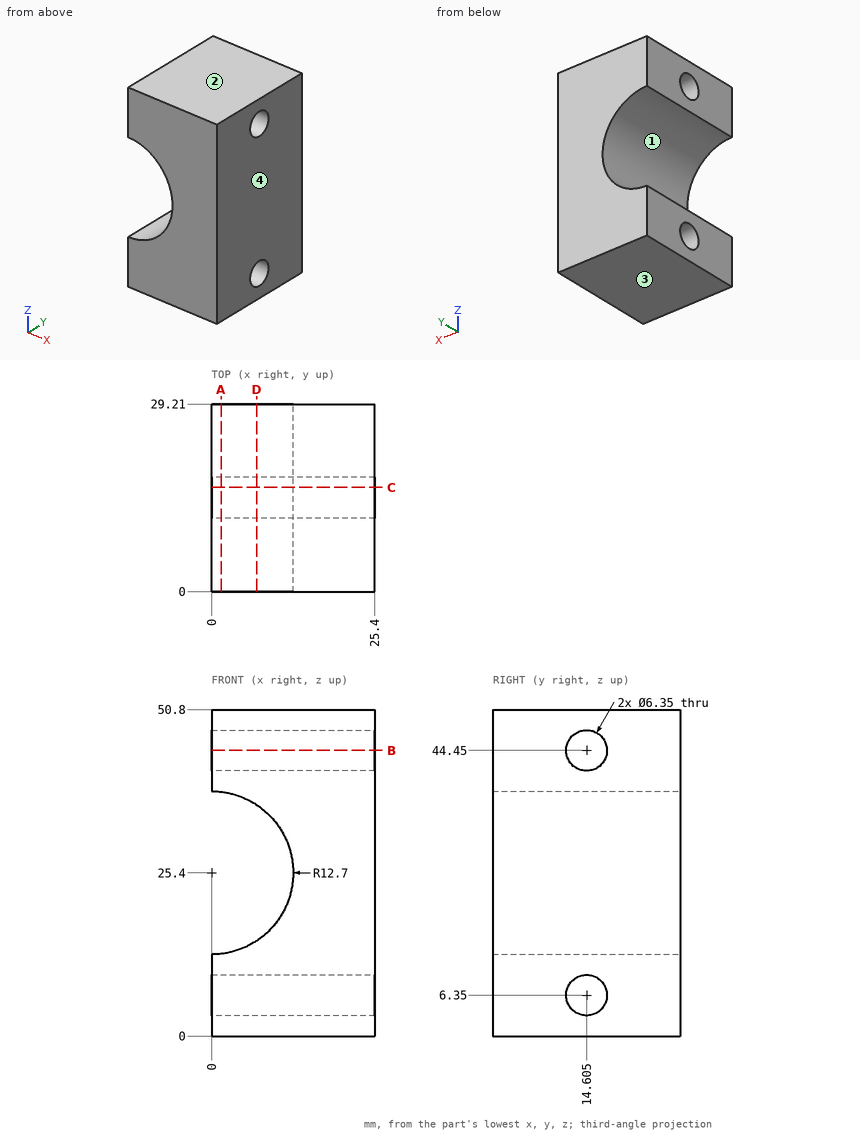
The drawing under review shows one solid part. Ordinate dimensions are in mm from its lowest x, y, z. Round coordinates to 2 decimals unless told otherwise and drop trailing zeros. Write each loop counter-clockwise with the first axis right and the second up, starting at its lowest first coordinate (ties: lowest second). Pieces come first, ordered by that corner, then holes. Notation, with made-up numbers: (13.5, 80) - (64.5, 80) arc R12 cw to (64.5, 101) - close; hole circle Ø1 at (-5.5, 74.25). An arc over 180 degrees is marked (long way). Put each result on its own line as item: value.
Q1. Mouldability with a two-part tool opening along Z and no side actions: class the marked faces 1, 2, 3 and 4 as released by +Z, released by -Z, zero draft, split by the parting line, or undercut.
Solved:
face 1: undercut
face 2: released by +Z
face 3: released by -Z
face 4: zero draft
Q2. We need section C-C (y = 16.25). Give the boundary of the cut face in (x, z).
Solved:
outline: (0, 0) - (25.4, 0) - (25.4, 3.63) - (0, 3.63) - close; (0, 9.07) - (25.4, 9.07) - (25.4, 41.73) - (0, 41.73) - (0, 38.1) arc R12.7 cw to (0, 12.7) - close; (0, 47.17) - (25.4, 47.17) - (25.4, 50.8) - (0, 50.8) - close
Q3. We need section D-D (x = 7). Give the boundary of the cut face in (y, z) (3 decimals), and give its area (3 significant figures).
Solved:
outline: (0, 0) - (29.21, 0) - (29.21, 14.803) - (0, 14.803) - close; (0, 35.997) - (29.21, 35.997) - (29.21, 50.8) - (0, 50.8) - close; hole circle Ø6.35 at (14.605, 6.35); hole circle Ø6.35 at (14.605, 44.45)
area: 801 mm2
Q4. Wall thickness on probe 1 along Z at (x, y) = (18.5, 13.75); probe 2 along Z at (x, y) = (18, 12.5); probe 3 along Z at (x, y) = (10, 14.5): over which ranges is each line inside the solid? List them lowest first.
Solved:
probe 1: z = 0 to 3.29, 9.41 to 41.39, 47.51 to 50.8
probe 2: z = 0 to 3.97, 8.73 to 42.07, 46.83 to 50.8
probe 3: z = 0 to 3.18, 9.52 to 17.57, 33.23 to 41.28, 47.62 to 50.8
Q5. We need section A-A (x = 1.5). Give the boundary of the cut face in (y, z) (3 decimals).
Solved:
outline: (0, 0) - (29.21, 0) - (29.21, 12.789) - (0, 12.789) - close; (0, 38.011) - (29.21, 38.011) - (29.21, 50.8) - (0, 50.8) - close; hole circle Ø6.35 at (14.605, 6.35); hole circle Ø6.35 at (14.605, 44.45)
Q6. We need section B-B (z = 44.45). Give the boundary of the cut face in (x, y), and give its area (3 significant figures).
Solved:
outline: (0, 0) - (25.4, 0) - (25.4, 11.43) - (0, 11.43) - close; (0, 17.78) - (25.4, 17.78) - (25.4, 29.21) - (0, 29.21) - close
area: 581 mm2
Q7. Insertion check: pin 1 Ø10 at (y, z) = (14.605, 44.45) entering from -X; pin 2 Ø1.5 at (y, z) = (23, 33.5) entering from -X; pin 3 Ø4 at (y, z) = (14.605, 6.35) entering from -X. Each pin has a flat end and moves straight along its axis. Give the tip position at first contact, or say it passes through.
Solved:
pin 1: stops at x = 0
pin 2: stops at x = 9.11
pin 3: passes through
